from build123d import *

# Parameters (mm, degrees)
F1_DEPTH = 25.0000008
F2_R     = 2.54
F3_DEPTH = 2.54
F4_R     = 2.54
F5_R     = 1.27


with BuildPart() as f1:
    # F0 (on Front) → F1 (new body)
    with BuildSketch(Plane.XZ):
        Polygon((-2.759046882, 29.6373917907), (-24.9089798809, 0), (55.0911141191, 0), align=None)
    extrude(amount=F1_DEPTH)

    # F2
    f2_edges = [f1.edges().sort_by_distance(p)[0] for p in [
        (-2.759047, -12.5, 29.637392),
    ]]
    fillet(f2_edges, radius=F2_R)

    # F3 (add): a face of the model
    f3_faces = [f1.faces().sort_by_distance(p)[0] for p in [
        (15.0910671191, -12.5000004, 0),
    ]]
    extrude(f3_faces, amount=F3_DEPTH)

    # F4
    f4_edges = [f1.edges().sort_by_distance(p)[0] for p in [
        (-24.90898, -12.5, 0),
    ]]
    fillet(f4_edges, radius=F4_R)

    # F5
    f5_edges = [f1.edges().sort_by_distance(p)[0] for p in [
        (55.091114, -12.5, 0),
    ]]
    fillet(f5_edges, radius=F5_R)


solid = f1.part
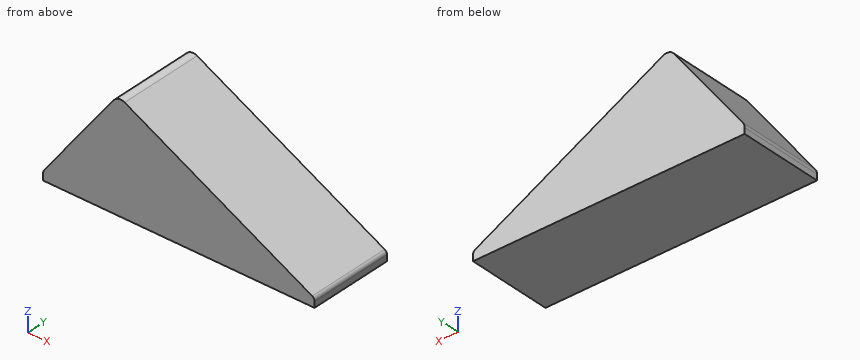
Here's how the part is built. I have some questions about the finished solid (model axes, mm). Give positions to 0.01 mm unless a question says otherwise; leave off trailing zeros. Loops run counter-clockwise (first coordinate to the right, second up) from the corner with the lowest first, then second, coordinate; pieces in that order, holes last. Notation, with made-up numbers: (-0.5, -30.5) -> (34.5, -30.5) arc R29 cw to (34.5, 0.5) -> close; hole circle Ø10 at (-1.75, 9). An arc over 180 degrees is marked (long way). Answer as a JSON object with one key per item and string values. Group by question number.
Item 1: I need wall thicknesses on L1, parallel to Z at x = 7, y = -14; L2, parallel to X at y = -3.5, z = 10; L3, parallel to Z at x = 50, y = -20. Which ranges of each line are inside material? Lowest first, please.
Item 2: Imagine slicing it at C-C on z = 4.5. Write out the boundary of the cut face in (x, y), then the cut area to 3 significant figures.
Item 3: Will this pin go through, and if not, where does the flat tip stop? pin 1 (1.5 mm diameter, centred on y = -8, z = 21, fed in from +X).
Item 4: Imagine slicing it at A-A on y = -21. Write out the boundary of the cut face in (x, z).
Item 5: Imagine slicing it at B-B on x = 7.5. Write out the boundary of the cut face in (y, z).
Answer list:
{
 "1": {"L1": "z = -2.54 to 24.64", "L2": "x = -17.44 to 35.57", "L3": "z = -2.54 to 2.61"},
 "2": {"outline": "(-21.55, -25) -> (46.31, -25) -> (46.31, 0) -> (-21.55, 0) -> close", "area": "1,700 mm2"},
 "3": {"pin 1": "stops at x = 15.56"},
 "4": {"outline": "(-24.91, -2.54) -> (55.09, -2.54) -> (55.09, -0.78) arc R1.27 ccw to (54.4, 0.35) -> (-0.85, 28.66) arc R2.54 ccw to (-4.04, 27.92) -> (-24.4, 0.68) arc R2.54 ccw to (-24.91, -0.84) -> close"},
 "5": {"outline": "(-25, -2.54) -> (0, -2.54) -> (0, 24.38) -> (-25, 24.38) -> close"}
}
